```python
from build123d import *

# Parameters (mm, degrees)
SKIZZE2_W                                   = 67
SKIZZE2_H                                   = 300
AUFSATZ_LINEAR_AUSTRAGEN1_DEPTH             = 2
FORMSENKUNG_F_R_M4_SENKSCHRAUBE_MIT_2_COUNT = 2
FORMSENKUNG_F_R_M4_SENKSCHRAUBE_MIT_2_PITCH = 270
SKIZZE9_W                                   = 31.10502621
SKIZZE9_H                                   = 6.710582317
SCHNITT_LINEAR_AUSTRAGEN5_DEPTH             = 10


with BuildPart() as part:
    # Skizze2 → Aufsatz-Linear austragen1 (new body)
    with BuildSketch(Plane.XY):
        with Locations((30.454545455, -53.853438228)):
            Rectangle(SKIZZE2_W, SKIZZE2_H)
    extrude(amount=AUFSATZ_LINEAR_AUSTRAGEN1_DEPTH)

    # Skizze4 → Formsenkung für M4 Senkschraube mit Innensechskant1 (revolve, cut)
    with BuildSketch(Plane(origin=(30.454545455, 81.146561772, 2), x_dir=(0, -1, 0), z_dir=(1, 0, 0))):
        Polygon((0, 0), (0, 2), (2.25, 2), (2.25, 2.05), (4.3, 0), align=None)
    formsenkung_f_r_m4_senkschraube_mit_inne = revolve(axis=Axis((30.454545455, 81.146561772, 8.35), (0, 0, -1)), mode=Mode.SUBTRACT)

    # Formsenkung f_r M4 Senkschraube mit  2: Formsenkung für M4 Senkschraube mit Innensechskant1 ×2
    with Locations(*[(0, -i * FORMSENKUNG_F_R_M4_SENKSCHRAUBE_MIT_2_PITCH, 0) for i in range(1, FORMSENKUNG_F_R_M4_SENKSCHRAUBE_MIT_2_COUNT)]):
        add(formsenkung_f_r_m4_senkschraube_mit_inne, mode=Mode.SUBTRACT)

    # Skizze9 → Schnitt-Linear austragen5 (cut)
    with BuildSketch(Plane.XY.offset(2)):
        Polygon((52.001558097, -91.692267967), (55.954864906, -99.53078632), (48.017183689, -102.940874601), (44.331709582, -95.41361182), align=None)
        with Locations((22.311332276, -97.288736457)):
            Rectangle(SKIZZE9_W, SKIZZE9_H)
        Polygon((6.758819171, -107.925887397), (50.350445865, -108.08808674), (50.427715289, -114.508189206), (23.217156686, -114.214287256), (37.758627479, -127.374767162), (37.758627479, -134.920795826), (24.5330538, -122.513026823), (6.876063428, -135.792670476), (6.986282299, -127.867340204), (20.398215233, -118.033810853), (17.474377356, -114.508189206), (6.841373177, -114.508189206), align=None)
        Polygon((32.81378197, -140.833783467), (37.956076493, -140.833783467), (37.863845381, -162.808656047), (33.104263457, -162.808656047), (12.007535601, -147.611290016), (12.007535601, -163.287666955), (6.986282299, -163.203737544), (6.986282299, -139.845285888), (11.322896284, -139.845285888), (32.81378197, -155.326589829), align=None)
        with BuildLine():
            Line((7.689666718, 25.787766367), (7.689666718, 18.106787224))
            Line((7.689666718, 18.106787224), (23.794942522, 18.106787224))
            add(Edge.make_bspline(
                [(23.794942522, 18.106787224), (32.601188558, 17.824016107), (32.801302406, 7.750150648)],
                knots=[0, 0, 0, 1, 1, 1], degree=2))
            Line((32.801302406, 7.750150648), (41.012907208, 7.750150648))
            add(Edge.make_bspline(
                [(35.769786279, 18.106787224), (41.216248983, 15.059838558), (41.012907208, 7.750150648)],
                knots=[0, 0, 0, 1, 1, 1], degree=2))
            Line((35.769786279, 18.106787224), (40.309969546, 18.106787224))
            Line((40.309969546, 18.106787224), (40.091631389, 25.787766367))
            Line((40.091631389, 25.787766367), (7.689666718, 25.787766367))
        make_face()
        with BuildLine():
            Line((28.488917876, -18.770250647), (31.817381195, -25.78965933))
            add(Edge.make_bspline(
                [(31.817381195, -25.78965933), (35.498176655, -24.019055478), (42.40530325, -18.074227702), (41.213657778, -2.009478612), (30.919016285, 4.141303213), (22.776211659, 4.831375661), (17.572864113, 3.89204048), (9.441685379, -0.413341636), (6.135963941, -7.921355494), (7.32226522, -18.888063748), (11.205018419, -23.673518651), (16.923657697, -26.06530754)],
                knots=[0, 0, 0, 0, 0.119409873, 0.27925359, 0.419931345, 0.450283778, 0.568056354, 0.605462622, 0.786940191, 0.828662398, 1, 1, 1, 1], degree=3))
            Line((16.923657697, -26.06530754), (20.431478316, -19.245299659))
            add(Edge.make_bspline(
                [(20.431478316, -19.245299659), (18.529961715, -18.448815365), (16.619467923, -17.425214119), (13.813302006, -13.511550753), (14.121204554, -6.483932431), (18.310146069, -4.418568869), (22.673204949, -3.485417269), (24.799039205, -3.418559428), (28.73741634, -3.960815369), (33.231832404, -6.011813728), (34.58703032, -11.56981876), (32.747718821, -16.344485846), (30.562040823, -18.053193176), (28.488917876, -18.770250647)],
                knots=[0, 0, 0, 0, 0.057281263, 0.077975222, 0.206939595, 0.4121179, 0.446671031, 0.540715366, 0.566135351, 0.689115335, 0.842004928, 0.873093394, 1, 1, 1, 1], degree=3))
        make_face()
        with BuildLine():
            Line((22.182559591, 55.683464558), (22.182559591, 31.646286217))
            add(Edge.make_bspline(
                [(22.182559591, 31.646286217), (28.285199554, 31.688242642), (36.493541258, 34.092996652), (40.550526158, 41.167443579), (41.105027709, 45.591258556)],
                knots=[0, 0, 0, 0, 0.555389856, 1, 1, 1, 1], degree=3))
            Line((41.105027709, 45.591258556), (34.50379781, 45.591258556))
            add(Edge.make_bspline(
                [(28.120055334, 40.440191437), (33.016316255, 40.899947408), (34.50379781, 45.591258556)],
                knots=[0, 0, 0, 1, 1, 1], degree=2))
            Line((28.120055334, 40.440191437), (28.120055334, 55.446553709))
            add(Edge.make_bspline(
                [(28.120055334, 55.446553709), (32.650059687, 54.608093435), (34.50379781, 50.422414638)],
                knots=[0, 0, 0, 1, 1, 1], degree=2))
            Line((34.50379781, 50.422414638), (41.104275737, 50.422414638))
            add(Edge.make_bspline(
                [(13.75926765, 31.756110501), (12.069853486, 33.007836098), (8.027031384, 37.003253409), (6.523132286, 43.013028309), (6.628333317, 56.311278281), (15.261430342, 63.498214031), (30.12062724, 65.215358583), (40.774477596, 58.523780449), (41.104275737, 50.422414638)],
                knots=[0, 0, 0, 0, 0.09000754, 0.234551371, 0.339423329, 0.540898393, 0.687756002, 1, 1, 1, 1], degree=3))
            Line((13.75926765, 31.756110501), (17.814541142, 38.76818417))
            add(Edge.make_bspline(
                [(17.814541142, 38.76818417), (15.599033207, 40.145840228), (13.917486025, 43.782276328), (14.533611479, 51.295203557), (17.892855837, 54.819575464), (22.182559591, 55.683464558)],
                knots=[0, 0, 0, 0, 0.22087745, 0.573734075, 1, 1, 1, 1], degree=3))
        make_face()
    extrude(amount=-SCHNITT_LINEAR_AUSTRAGEN5_DEPTH, mode=Mode.SUBTRACT)


solid = part.part
```
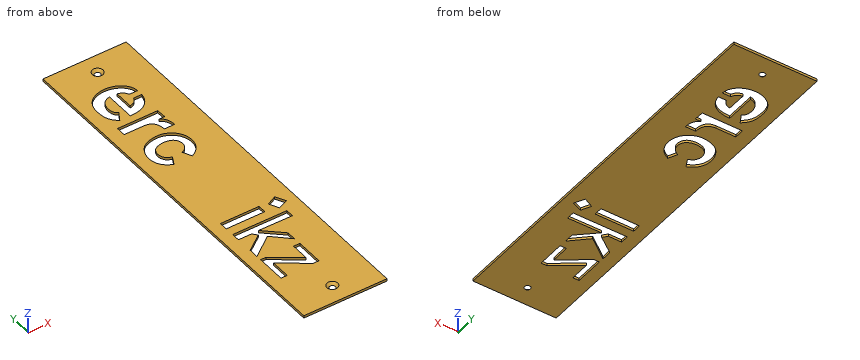
Could you check a few things on this model? Use its own coordinates, in mm. Coordinates: 2 decimals unless noted, no trailing zeros. Write each loop counter-clockwise with the first axis right and the second up, starting at its lowest first coordinate (ties: lowest second). Pieces come first, ordered by that corner, then holes. Notation, with made-up numbers: M 15,83 L 55,83 A17 cw 55,116 Z; hole C 28,63 d4. An arc over 180 degrees is marked long. Answer as CSV lines item,"result". Start each with the question number.
1) I want a section at A-A, the plane y = -159. Please give me the cut outline in (x, z).
2) Please list where these lines run through material, in increasing order: line 1 (X direction, y = 46, z = 0.2); line 2 (X direction, y = -13, z = 1.35); line 3 (X direction, y = -153.5, z = 1.1). Write a range as from..to.
3) I want a section at B-B, the plane z = 0.6. Give the number of separate pieces and of enclosed holes in the cut face, and give its area (3 significant figures).
Data:
1,outline,"M -3.05,0 L 6.99,0 L 6.99,2 L -3.05,2 Z; M 12.01,0 L 27.82,0 L 27.82,2 L 12.01,2 Z; M 37.88,0 L 63.95,0 L 63.95,2 L 37.88,2 Z"
2,line 1,"x = -3.05..6.67, 14.3..22.18, 28.12..63.95"
2,line 2,"x = -3.05..6.73, 14.3..33.91, 41.24..63.95"
2,line 3,"x = -3.05..6.99, 12.01..20.18, 30.28..32.81, 37.9..63.95"
3,separate pieces,"1"
3,enclosed holes,"9"
3,area,"17,300 mm^2"
